```python
from build123d import *

# Parameters (mm, degrees)
SKETCH1_W           = 76.2
SKETCH1_H           = 101.6
BOSS_EXTRUDE1_DEPTH = 1143
SKETCH2_W           = 63.5
SKETCH2_H           = 88.9
CUT_EXTRUDE1_DEPTH  = 1145.76252996
SKETCH3_R           = 8.89
CUT_EXTRUDE2_DEPTH  = 1147.663019374


with BuildPart() as part:
    # Sketch1 → Boss-Extrude1 (new body)
    with BuildSketch(Plane(origin=(0, 0, 0), x_dir=(1, 0, 0), z_dir=(0, 1, 0))):
        Rectangle(SKETCH1_W, SKETCH1_H)
    extrude(amount=-BOSS_EXTRUDE1_DEPTH)

    # Sketch2 → Cut-Extrude1 (cut, through all)
    with BuildSketch(Plane.XZ.offset(1143)):
        Rectangle(SKETCH2_W, SKETCH2_H)
    extrude(amount=-CUT_EXTRUDE1_DEPTH, mode=Mode.SUBTRACT)

    # Sketch3 → Cut-Extrude2 (cut, through all)
    with BuildSketch(Plane(origin=(38.1, 0, 0), x_dir=(0, 0, -1), z_dir=(1, 0, 0))):
        with Locations((0, -996.95)):
            Circle(SKETCH3_R)
        with Locations((0, -819.15)):
            Circle(SKETCH3_R)
    extrude(amount=-CUT_EXTRUDE2_DEPTH, mode=Mode.SUBTRACT)


solid = part.part
```
Source: CAD feature listing. Evaluate the final solid. Frame: model axes, mm. A direction names the side the tool comes from. Give positions to 0.01 mm unless a question says otherwise; leave off trailing zeros. Order: outer loops, then holes, each group sorted by start corner. A loop starts at its lowest first (then second) coordinate and runs counter-clockwise, first axis right, second up. Notation, with made-up numbers: (-2, 31.5) -> (57, 31.5) arc R21 cw to (57, 36.5) -> close; hole circle Ø9 at (-11, 64). An arc over 180 degrees is marked (long way). Use a Markdown table: item, result.
Q1. Section B-B (y = -747). Return the cut outline in (x, z), and give its area (3 significant figures).
A:
| item | result |
|---|---|
| outline | (-38.1, -50.8) -> (38.1, -50.8) -> (38.1, 50.8) -> (-38.1, 50.8) -> close; hole (-31.75, -44.45) -> (31.75, -44.45) -> (31.75, 44.45) -> (-31.75, 44.45) -> close |
| area | 2,100 mm^2 |
Q2. Access query for faces 4 (the face through (0, -580, -44.45)), 5 (the face through (38.1, -563, 1)). Directions: +Z, -Z, +X, -X, +Y, -Y. A direction counts if a zero-diameter tool reaches every point of the face in a straight line with its end or side. Return the directions, or none.
A:
| item | result |
|---|---|
| face 4 | +Y, -Y |
| face 5 | +Z, -Z, +X, +Y, -Y |
Q3. Material intervals for line 1 (Y direction, x = 35, z = 0); line 2 (Z direction, x = -25.5, y = -241.5); line 3 (X direction, y = -602, z = -40.5), sorted ascending. Write a range as [from, to].
A:
| item | result |
|---|---|
| line 1 | [-1143, -1005.84], [-988.06, -828.04], [-810.26, 0] |
| line 2 | [-50.8, -44.45], [44.45, 50.8] |
| line 3 | [-38.1, -31.75], [31.75, 38.1] |
Q4. First-contact query: P1, Ø10.5, axis at y = -996.95, z = 0, coming from the -X side. Flat tip, straight axial feed; report the tip coordinate or a pass-through.
A:
| item | result |
|---|---|
| P1 | through |
Q5. Pull-direction query (Y, two-part tool) for faces 1 (the face through (34.97, -1005.63, 1.93)), 2 (the face through (-38.1, -563, 1)), 3 (the face through (-34, -1143, 0)); classes: +Y half, -Y half, draft (parallel to the pull), parting line (faces both ways), or undercut.
A:
| item | result |
|---|---|
| face 1 | undercut |
| face 2 | draft |
| face 3 | -Y half |
Q6. Section A-A (x = -1). Return the cut outline in (y, z), and give its area (3 significant figures).
A:
| item | result |
|---|---|
| outline | (-1143, -50.8) -> (0, -50.8) -> (0, -44.45) -> (-1143, -44.45) -> close; (-1143, 44.45) -> (0, 44.45) -> (0, 50.8) -> (-1143, 50.8) -> close |
| area | 14,500 mm^2 |
